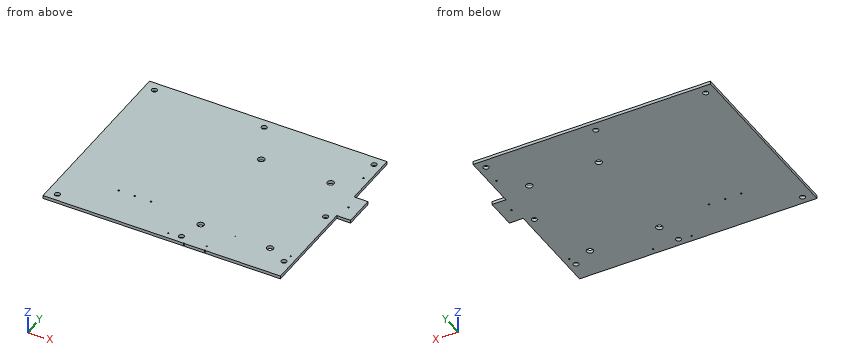
Solid Edge part; units mm, degrees
sketch "Sketch1" plane through (0, 0, 0) normal (0, 0, 1) x (1, 0, 0)
  line L0 (-105, -61.5) -> (105, -61.5)
  line L1 (105, -61.5) -> (105, 61.5)
  line L2 (105, 61.5) -> (-105, 61.5)
  line L3 (-105, 61.5) -> (-105, -61.5)
  dimension "D1" = 105
  dimension "D2" = 105
extrude "Protrusion1" add sketch "Sketch1" along normal blind 2
hole "Hole1" at (-1, -57.5, 2) direction (0, 0, -1) diameter 0.8 end through all
hole "Hole2" at (-26, -57.5, 2) direction (0, 0, -1) diameter 0.8 end through all
sketch "Sketch2" plane through (0, 0, 2) normal (0, 0, 1) x (-1, 0, 0)
  line L0 (-0.25, 61) -> (0.25, 61)
  line L1 (0.25, 61) -> (0.25, 61.5)
  line L2 (0.25, 61.5) -> (-0.25, 61.5)
  line L3 (-0.25, 61.5) -> (-0.25, 61)
  dimension "D1" = 0.25
extrude "Cutout1" cut sketch "Sketch2" against normal through all
sketch "Sketch3" plane through (0, 0, 2) normal (0, 0, 1) x (1, 0, 0)
  line L0 (105, -61.5) -> (105, 61.5)
  line L1 (49, -61.5) -> (105, -61.5)
  line L2 (49, 3.5) -> (49, -61.5)
  line L3 (58, 3.5) -> (49, 3.5)
  line L4 (58, 23.5) -> (58, 3.5)
  line L5 (49, 23.5) -> (58, 23.5)
  line L6 (49, 61.5) -> (49, 23.5)
  line L7 (105, 61.5) -> (49, 61.5)
  dimension "D1" = 58
  dimension "D2" = 49
  dimension "D3" = 49
extrude "Ausschnitt_3" cut sketch "Sketch3" against normal blind 2
hole "Hole3" at (-98.5, 55.5, 2) direction (0, 0, -1) diameter 3.5 end through all
hole "Hole4" at (44, 55.5, 2) direction (0, 0, -1) diameter 3.5 end through all
hole "Hole5" at (44, -48.5, 2) direction (0, 0, -1) diameter 3.5 end through all
hole "Hole6" at (-18, -56.5, 2) direction (0, 0, -1) diameter 3.5 end through all
hole "Hole7" at (-98.5, -56.5, 2) direction (0, 0, -1) diameter 3.5 end through all
hole "Hole8" at (44, -0.5, 2) direction (0, 0, -1) diameter 3.5 end through all
hole "Hole9" at (-27.25, 55.5, 2) direction (0, 0, -1) diameter 3.5 end through all
hole "Hole10" at (45, -42.5, 2) direction (0, 0, -1) diameter 1 end through all
hole "Hole11" at (45, 41.5, 2) direction (0, 0, -1) diameter 1 end through all
hole "Hole12" at (51, 13.5, 2) direction (0, 0, -1) diameter 1 end through all
hole "Hole13" at (-59.5, -36.5, 2) direction (0, 0, -1) diameter 1 end through all
hole "Hole14" at (-49, -36.5, 2) direction (0, 0, -1) diameter 1 end through all
hole "Hole15" at (-70, -36.5, 2) direction (0, 0, -1) diameter 1 end through all
hole "Hole16" at (31, 28.5, 2) direction (0, 0, -1) diameter 4.3 end up to next
hole "Hole17" at (31, -41.5, 2) direction (0, 0, -1) diameter 4.3 end up to next
hole "Hole18" at (-14, -41.5, 2) direction (0, 0, -1) diameter 4.3 end up to next
hole "Hole19" at (-14, 28.5, 2) direction (0, 0, -1) diameter 4.3 end up to next
hole "Hole20" at (8.5, -41.5, 2) direction (0, 0, -1) diameter 0.2 end through all
hole "Hole21" at (8.5, 28.5, 2) direction (0, 0, -1) diameter 0.2 end through all
sketch "Sketch4" plane through (-23.4888, 0, 2) normal (0, 0, 1) x (1, 0, 0)
  line L0 (9.7388, -61.5) -> (10.2388, -61.5)
  line L1 (10.2388, -61.5) -> (10.2388, -61)
  line L2 (10.2388, -61) -> (9.7388, -61)
  line L3 (9.7388, -61) -> (9.7388, -61.5)
  dimension "D1" = 10.2388
extrude "Cutout2" cut sketch "Sketch4" against normal through all
Input: part model. Units: mm. Frame: model coordinates. Round coordinates to 2 decimals unless told otherwise and drop trailing zeros. Write each loop counter-clockwise with the first axis right and the second up, starting at its lowest first coordinate (ties: lowest second). Pieces come first, ordered by that corner, then holes.
1) Cut plane D-D (z = 1.65). Count the separate pieces of the cut face and the enclosed holes in it, then the cut area to 3 significant figures.
2) Cut plane B-B (y = -0.5). Return the cut outline in (x, z), then the cut area to 3 significant figures.
3) Contact query for flat-ended pins moving along their axis: P1, Ø0.6, axis at x = 54.5, z = 1.5, coming from the -Y side; P2, Ø0.6, axis at y = -13.5, z = 1.5, coming from the +X side. Output: stop coordinate, or through.
4) Ray query, L1, parallel to Y at x = -14, z = 1.1; L2, parallel to Y at x = 44, z = 0.9; L3, parallel to X at y = 28.5, z = 0.95. Return the intervals inside material, ascending.
5) Cut plane A-A (x = 31). Return the cut outline in (y, z), then the cut area to 3 significant figures.
6) Cut plane C-C (y = 55.5). Return the cut outline in (x, z).
Geometry says:
1. separate pieces: 1
1. enclosed holes: 21
1. area: 19,000 mm2
2. outline: (-105, 0) - (42.25, 0) - (42.25, 2) - (-105, 2) - close; (45.75, 0) - (49, 0) - (49, 2) - (45.75, 2) - close
2. area: 301 mm2
3. P1: stops at y = 3.5
3. P2: stops at x = 49
4. L1: y = -61.5 to -43.65, -39.35 to 26.35, 30.65 to 61.5
4. L2: y = -61.5 to -50.25, -46.75 to -2.25, 1.25 to 53.75, 57.25 to 61.5
4. L3: x = -105 to -16.15, -11.85 to 8.4, 8.6 to 28.85, 33.15 to 49
5. outline: (-61.5, 0) - (-43.65, 0) - (-43.65, 2) - (-61.5, 2) - close; (-39.35, 0) - (26.35, 0) - (26.35, 2) - (-39.35, 2) - close; (30.65, 0) - (61.5, 0) - (61.5, 2) - (30.65, 2) - close
5. area: 229 mm2
6. outline: (-105, 0) - (-100.25, 0) - (-100.25, 2) - (-105, 2) - close; (-96.75, 0) - (-29, 0) - (-29, 2) - (-96.75, 2) - close; (-25.5, 0) - (42.25, 0) - (42.25, 2) - (-25.5, 2) - close; (45.75, 0) - (49, 0) - (49, 2) - (45.75, 2) - close
